Autodesk Fusion 360 part; units mm, degrees
sketch "Sketch1" plane through (0, 0, 0) normal (1, 0, 0) x (0, 1, 0)
  line L0 (3.2, 17) -> (8, 11)
  line L1 (8, 11) -> (5, 11)
  line L2 (0, 17) -> (3.2, 17)
  line L3 (5, 11) -> (5, 5) construction
  line L4 (0, 17) -> (5, 9.0465) construction
  line L5 (20, 0) -> (0, 0)
  line L6 (5, 5) -> (1.5967, 14.4602)
  line L7 (0, 0) -> (0, 21) construction
  line L8 (0, 21) -> (8, 11) construction
  line L9 (5, 5) -> (20, 5)
  line L10 (0, 0) -> (0, 17)
  line L11 (1.5967, 14.4602) -> (5, 11)
  line L12 (2.1849, 12.8252) -> (2.8151, 13.2214) construction
  line L13 (20, 0) -> (20, 5)
  dimension "d4" = 20
  dimension "d5" = 8
  dimension "d6" = 5
  dimension "d7" = 21
  dimension "d8" = 6
  dimension "d9" = 5
  dimension "d25" = 17
  dimension "d26" = 3
extrude "Extrude1" add sketch "Sketch1" along normal blind 5
fillet "Fillet1" radius 1 5 edges at (2.5, 3.2, 17) (2.5, 0, 17) (2.5, 0, 0) (2.5, 5, 11) (2.5, 8, 11)
fillet "Fillet2" radius 0.5 1 edges at (2.5, 1.5967, 14.4602)
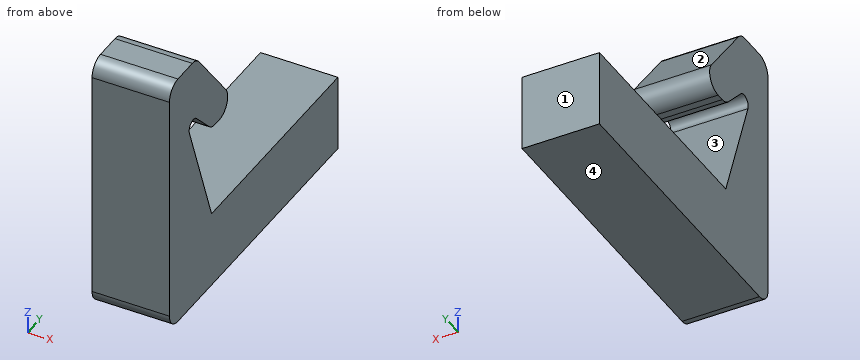
Input: part model. Units: mm. Frame: model coordinates. Face numbers are marked on the shaded views. Give positions to 0.01 mm unless a question says otherwise; leave off trailing zeros. Order: outer loops, then holes, each group sorted by start corner. A loop starts at its lowest first (then second) coordinate and runs counter-clockwise, first axis right, second up. Notation, with made-up numbers: (3.25, 65) - (58.25, 65) arc R12 ccw to (58.25, 87) - close; hole circle Ø2 at (80, -10). An arc over 180 degrees is marked (long way). Use a Markdown table: item, result.
(1) Pin query (flat end, axial travel): pin 1 (2.5 mm diameter, centred on x = 2, y = 11, fed in from +Z); pin 2 (1 mm diameter, centred on x = 2, z = 15, fed in from +Y). Return the tip coordinate at first contact, or that it passes through.
Computed values:
| item | result |
|---|---|
| pin 1 | stops at z = 5 |
| pin 2 | stops at y = 5.2 |
(2) Section query A-A (x = 0.9). Output: boundary loops of the cut face in (y, z), then the cut area to 3 significant figures.
Computed values:
| item | result |
|---|---|
| outline | (0, 1) arc R1 ccw to (1, 0) - (20, 0) - (20, 5) - (5, 5) - (2.37, 12.31) arc R0.5 cw to (3.2, 12.83) - (4.71, 11.3) arc R1 ccw to (5.42, 11) - (5.92, 11) arc R1 ccw to (6.7, 12.62) - (3.5, 16.62) arc R1 ccw to (2.72, 17) - (1, 17) arc R1 ccw to (0, 16) - close |
| area | 153 mm2 |
(3) Draft query along Z for the marked faces 1, 2, 3 and 4. Return one class per face: released by +Z, released by -Z, zero draft, split by the parting line, or undercut.
Computed values:
| item | result |
|---|---|
| face 1 | zero draft |
| face 2 | released by +Z |
| face 3 | undercut |
| face 4 | released by -Z |
(4) Section query B-B (z = 15.75). Output: boundary loops of the cut face in (x, y).
Computed values:
| item | result |
|---|---|
| outline | (0, 0) - (5, 0) - (5, 4.2) - (0, 4.2) - close |
(5) Section query C-C (y = 10). Output: boundary loops of the cut face in (x, z), then the cut area to 3 significant figures.
Computed values:
| item | result |
|---|---|
| outline | (0, 0) - (5, 0) - (5, 5) - (0, 5) - close |
| area | 25.0 mm2 |
(6) Line query: line 1 (Y direction, x = 2.7, z = 14.75); line 2 (Z direction, x = 3.05, y = 6.25). Output: solid intervals per line, ascending. Write a range as from..to.
Computed values:
| item | result |
|---|---|
| line 1 | y = 0..5 |
| line 2 | z = 0..5, 11.06..13.19 |
